The listing builds one solid part. Answer for the finished solid, in the listing's coordinates (mm). Coordinates: 2 decimals unless noted, no trailing zeros. Loops run counter-clockwise (first coordinate to the right, second up) from the corner with the lowest first, then second, coordinate; pieces in that order, holes last. Notation, with made-up numbers: (0.5, 10) - (24.5, 10) arc R24 ccw to (24.5, 45) - close; hole circle Ø5 at (18.5, 84). An arc over 180 degrees is marked (long way). Use one line per item in the form item = value. Start each with the question number.
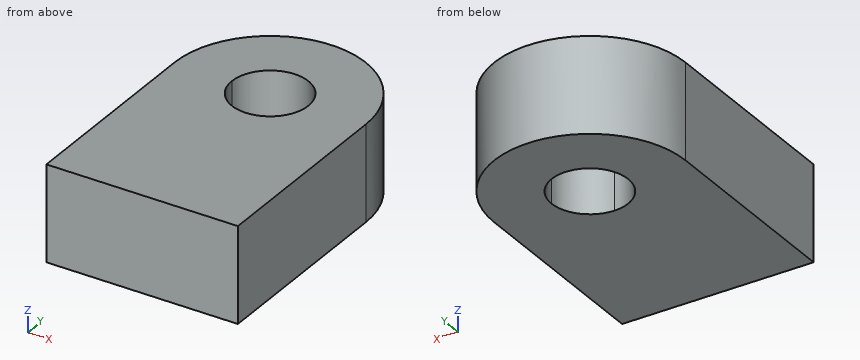
```python
from build123d import *

# Parameters (mm, degrees)
EXTRUDE_1_DEPTH = 10


with BuildPart() as part:
    # 스케치1 → 보스-돌출1 (new body)
    with BuildSketch(Plane.XY):
        with BuildLine():
            ThreePointArc((10, 21), (0, 31), (-10, 21))
            Line((-10, 21), (-4, 21))
            ThreePointArc((-4, 21), (0, 25), (4, 21))
            Line((4, 21), (10, 21))
        make_face()
        with BuildLine():
            ThreePointArc((-10, 21), (-7.071067812, 13.928932188), (0, 11))
            Line((0, 11), (0, 17))
            ThreePointArc((0, 17), (-2.828427125, 18.171572875), (-4, 21))
            Line((-4, 21), (-10, 21))
        make_face()
        with BuildLine():
            Line((0, 17), (0, 11))
            ThreePointArc((0, 11), (7.071067812, 13.928932188), (10, 21))
            Line((10, 21), (4, 21))
            ThreePointArc((4, 21), (2.828427125, 18.171572875), (0, 17))
        make_face()
        with BuildLine():
            Line((0, 11), (0, 0))
            Line((0, 0), (10, 0))
            Line((10, 0), (10, 21))
            ThreePointArc((10, 21), (7.071067812, 13.928932188), (0, 11))
        make_face()
        with BuildLine():
            Line((-10, 0), (0, 0))
            Line((0, 0), (0, 11))
            ThreePointArc((0, 11), (-7.071067812, 13.928932188), (-10, 21))
            Line((-10, 21), (-10, 0))
        make_face()
    extrude(amount=EXTRUDE_1_DEPTH)


solid = part.part
```
(1) Find the intervals of material crossed by probe 1 along Y at (x, z) = (2.5, 6.5); probe 2 along Y at (x, z) = (-1.5, 7.5); probe 3 along Y at (x, z) = (-4.75, 4.75), in increasing order. Write a range as from..to.
(2) A cutting plane is placed at B-B (z = 4.5). Determine the outline of the cut face in (x, y).
(3) A cutting plane is placed at A-A (x = -2.5). Determine the outline of the cut face in (y, z).
(4) A cutting plane is placed at D-D (x = 1.5). Determine the outline of the cut face in (y, z).
(5) A cutting plane is placed at C-C (y = 27). Determine the outline of the cut face in (x, z).
(6) Each of these flat-tipped pins is pushed along its axis until it touches: pin 1 Ø3 at (x, z) = (2, 7.5) entering from +Y; pin 2 Ø1.5 at (y, z) = (27, 4.5) entering from -X. Where does it stop, or does it pass through?
Evaluation:
q1.probe_1 = 0..17.88, 24.12..30.68
q1.probe_2 = 0..17.29, 24.71..30.89
q1.probe_3 = 0..29.8
q2.outline = (-10, 0) - (10, 0) - (10, 21) arc R10 ccw to (-10, 21) - close; hole circle Ø8 at (0, 21)
q3.outline = (0, 0) - (17.88, 0) - (17.88, 10) - (0, 10) - close; (24.12, 0) - (30.68, 0) - (30.68, 10) - (24.12, 10) - close
q4.outline = (0, 0) - (17.29, 0) - (17.29, 10) - (0, 10) - close; (24.71, 0) - (30.89, 0) - (30.89, 10) - (24.71, 10) - close
q5.outline = (-8, 0) - (8, 0) - (8, 10) - (-8, 10) - close
q6.pin_1 = 30.99
q6.pin_2 = -8.51
